Check sheet for the modelled part. Datum: model origin and axes. Units: mm. Face numbers are marked on the shaded views. A direction names the side the tool comes from. Round coordinates to 2 decimals unless told otherwise and drop trailing zeros. Write each loop counter-clockwise with the first axis right and the second up, starting at its lowest first coordinate (ties: lowest second). Pieces come first, ordered by that corner, then holes.
Item 1: Cross-section at C-C on z = 18.5. Enter the section's corners in (x, y), plus the area to 3 significant figures.
Item 2: Material ranges on line 1 (Y direction, x = 1.25, z = 10); line 2 (Z direction, x = 1.5, y = 74.5); line 3 (X direction, y = 117, z = 15), recorded low to high.
Item 3: Tool access check on the marked faces 4 and 5. Record the directions out of +Z, -Z, +X, -X, +Y, -Y that give a thin tool (end or side, any length) a straight path to the whole face; none if there is none.
Item 4: Go/stop test with flat-tipped pins: pin 1 Ø2 at (y, z) = (180.5, 25) entering from -X; pin 2 Ø10 at (x, y) = (15, 59.5) entering from -Z; pin 3 Ø7.5 at (x, z) = (-0.5, 18) entering from +Y; pin 4 Ø7.5 at (y, z) = (187.5, 10.5) entering from -X. Record where each tip stops, or that it passes through.
Item 5: Cross-section at A-A on y = 78. Enter the section's corners in (x, z).
Item 6: Release check for a two-part mould opening along Z. For the marked faces 1, 2 and 3 record: +Z half, -Z half, draft (parallel to the pull), parting line (faces both ways), or undercut.
Item 7: Cross-section at B-B on z = 64. Enter the section's corners in (x, y), plus the area to 3 significant figures.
from build123d import *

# Parameters (mm, degrees)
BOSS_EXTRUDE1_DEPTH     = 30
SKETCH2_R               = 17.5
BOSS_EXTRUDE2_DEPTH     = 60
BOSS_EXTRUDE3_DEPTH     = 350
CUT_EXTRUDE1_DEPTH      = 387.910842443
CUT_EXTRUDE1_DEPTH_BACK = 350
SKETCH4_R               = 7.5
SKETCH5_W               = 10
SKETCH5_H               = 10
BOSS_EXTRUDE4_DEPTH     = 15
SKETCH6_R               = 3
CUT_EXTRUDE2_DEPTH      = 388.201497931


with BuildPart() as part:
    # Sketch1 → Boss-Extrude1 (new body)
    with BuildSketch(Plane(origin=(0, 0, 0), x_dir=(1, 0, 0), z_dir=(0, 1, 0))):
        with BuildLine():
            Line((-20, -50), (-20, 0))
            Line((-20, 0), (20, 0))
            Line((20, 0), (20, -50))
            ThreePointArc((20, -50), (0, -70), (-20, -50))
        make_face()
    extrude(amount=BOSS_EXTRUDE1_DEPTH)

    # Sketch2 → Boss-Extrude2 (add)
    with BuildSketch(Plane(origin=(0, 30, 0), x_dir=(1, 0, 0), z_dir=(0, 1, 0))):
        with Locations(Location((0, -50, 0), (0, 0, 90))):
            Circle(SKETCH2_R)
    extrude(amount=BOSS_EXTRUDE2_DEPTH)

    # Sketch3 → Boss-Extrude3 (add)
    with BuildSketch(Plane(origin=(0, 30, 0), x_dir=(1, 0, 0), z_dir=(0, 1, 0))):
        with BuildLine():
            Line((-12.5, 0), (-12.5, -15))
            ThreePointArc((-12.5, -15), (0, -27.5), (12.5, -15))
            Line((12.5, -15), (12.5, 0))
            Line((12.5, 0), (-12.5, 0))
        make_face()
    extrude(amount=BOSS_EXTRUDE3_DEPTH)

    # Sketch4 → Cut-Extrude1 (cut, two sides: drawn at the far end of the back side and taken through both)
    with BuildSketch(Plane(origin=(0, 380, 0), x_dir=(1, 0, 0), z_dir=(0, 1, 0)).offset(-CUT_EXTRUDE1_DEPTH_BACK)):
        with Locations(Location((0, -15, 0), (0, 0, 90))):
            Circle(SKETCH4_R)
    extrude(amount=CUT_EXTRUDE1_DEPTH + CUT_EXTRUDE1_DEPTH_BACK, mode=Mode.SUBTRACT)

    # Sketch5 → Boss-Extrude4 (add)
    with BuildSketch(Plane(origin=(0, 0, 0), x_dir=(-1, 0, 0), z_dir=(0, -1, 0))):
        with Locations((0, -10)):
            Rectangle(SKETCH5_W, SKETCH5_H)
    extrude(amount=BOSS_EXTRUDE4_DEPTH)

    # Sketch6 → Cut-Extrude2 (cut, through all)
    with BuildSketch(Plane(origin=(5, 0, 0), x_dir=(0, 0, -1), z_dir=(1, 0, 0))):
        with Locations((-10, -10)):
            Circle(SKETCH6_R)
    extrude(amount=-CUT_EXTRUDE2_DEPTH, mode=Mode.SUBTRACT)


solid = part.part
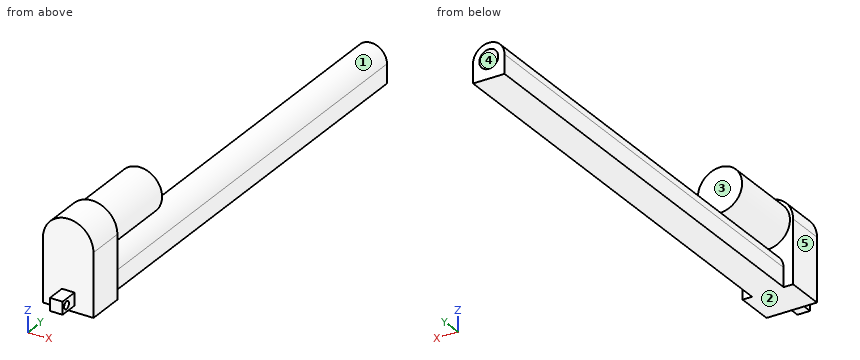
Response values:
1. outline: (-20, 0) - (20, 0) - (20, 30) - (12, 30) - (12, 380) - (6.63, 380) - (6.63, 30) - (-6.63, 30) - (-6.63, 380) - (-12, 380) - (-12, 30) - (-20, 30) - close
1. area: 4,960 mm2
2. line 1: y = -15 to -13, -7 to 30
2. line 2: z = 0 to 7.65, 22.35 to 27.41, 32.56 to 67.44
2. line 3: x = -12.5 to -7.5, 7.5 to 12.5
3. face 4: +Y
3. face 5: +Z, -Z, -X, +Y, -Y
4. pin 1: stops at x = -8.67
4. pin 2: stops at z = 0
4. pin 3: stops at y = 30
4. pin 4: stops at x = -12.5
5. outline: circle Ø35 at (0, 50); (-12.5, 0) - (12.5, 0) - (12.5, 15) arc R12.5 ccw to (-12.5, 15) - close; hole circle Ø15 at (0, 15)
6. face 1: undercut
6. face 2: -Z half
6. face 3: draft
7. outline: (-14.28, 0) - (14.28, 0) - (14.28, 30) - (10.5, 30) - (10.5, 90) - (-10.5, 90) - (-10.5, 30) - (-14.28, 30) - close
7. area: 2,120 mm2
